from build123d import *

# Parameters (mm, degrees)
F0_W     = 48.26
F0_H     = 45.72
F0_R     = 1.397
F0_R_2   = 3.175
F1_DEPTH = 60.96
F2_DEPTH = 12.7
F3_DEPTH = 7.62


with BuildPart() as f1:
    # F0 (on Top) → F1 (new body)
    with BuildSketch(Plane.XY):
        Rectangle(F0_W, F0_H)
        with Locations((-17.145, -15.875)):
            Circle(F0_R, mode=Mode.SUBTRACT)
        with Locations((0, -15.875)):
            Circle(F0_R_2, mode=Mode.SUBTRACT)
        with Locations((17.145, -15.875)):
            Circle(F0_R, mode=Mode.SUBTRACT)
        with Locations((-17.145, 15.875)):
            Circle(F0_R, mode=Mode.SUBTRACT)
        with Locations((0, 15.875)):
            Circle(F0_R_2, mode=Mode.SUBTRACT)
        with Locations((17.145, 15.875)):
            Circle(F0_R, mode=Mode.SUBTRACT)
        with Locations((0, 15.875)):
            Circle(F0_R_2)
        with Locations((0, -15.875)):
            Circle(F0_R_2)
        with Locations((-17.145, 15.875)):
            Circle(F0_R)
        with Locations((-17.145, -15.875)):
            Circle(F0_R)
        with Locations((17.145, 15.875)):
            Circle(F0_R)
        with Locations((17.145, -15.875)):
            Circle(F0_R)
    extrude(amount=-F1_DEPTH)

    # F0 (on Top) → F2 (cut)
    with BuildSketch(Plane.XY):
        with Locations((-17.145, 15.875)):
            Circle(F0_R)
        with Locations((-17.145, -15.875)):
            Circle(F0_R)
        with Locations((17.145, 15.875)):
            Circle(F0_R)
        with Locations((17.145, -15.875)):
            Circle(F0_R)
    extrude(amount=-F2_DEPTH, mode=Mode.SUBTRACT)

    # F0 (on Top) → F3 (join)
    with BuildSketch(Plane.XY):
        with Locations((0, 15.875)):
            Circle(F0_R_2)
        with Locations((0, -15.875)):
            Circle(F0_R_2)
    extrude(amount=F3_DEPTH)


solid = f1.part
Read the model definition and answer for the solid it produces. Units are mm, in the model's axes. A direction names the side the tool comes from. Coordinates: 2 decimals unless noted, no trailing zeros. Loops run counter-clockwise (first coordinate to the right, second up) from the corner with the lowest first, then second, coordinate; pieces in that order, holes last.
Q1. The part is cut by section B-B on y = 6. Write down the section's boundary in (x, z).
Q2. The part is cut by section A-A on x = 0. Write down the section's boundary in (y, z).
Q3. The mould has two halves that part along X. Classify faces 1 (the face through (-24.13, 0, -30)), 2 (the face through (0, -16, 7.62)), 3 (the face through (17, -16, -12.7)): +X half, -X half, draft (parallel to the pull), parting line (faces both ways), or undercut.
Q4. Consider probe 1 along Z at (x, y) = (17, -14); probe 2 along X at (y, z) = (13, 1.5). Determine where each line is inside the solid, lowest interval first.
Q5. Each of these flat-tipped pins is pushed along its axis until it touches: pin 1 Ø6 at (x, y) = (-9.5, -5.5) entering from +Z; pin 2 Ø0.8 at (x, y) = (17, -15.5) entering from +Z. Where does it stop, or does it pass through?
Q6. Which of the six approach directions +Z, -Z, +X, -X, +Y, -Y give full straight-line access (tool end or side, diameter ignored) to faces 4 (the face through (0, 16, 7.62)), 5 (the face through (-0.413, 19.023, 3.757))?
Q7. The part is cut by section C-C on x = -10.5. Write down the section's boundary in (y, z).
Results below:
1. outline: (-24.13, -60.96) - (24.13, -60.96) - (24.13, 0) - (-24.13, 0) - close
2. outline: (-22.86, -60.96) - (22.86, -60.96) - (22.86, 0) - (19.05, 0) - (19.05, 7.62) - (12.7, 7.62) - (12.7, 0) - (-12.7, 0) - (-12.7, 7.62) - (-19.05, 7.62) - (-19.05, 0) - (-22.86, 0) - close
3. face 1: -X half
3. face 2: draft
3. face 3: undercut
4. probe 1: z = -60.96 to 0
4. probe 2: x = -1.35 to 1.35
5. pin 1: stops at z = 0
5. pin 2: stops at z = -12.7
6. face 4: +Z, +X, -X, +Y, -Y
6. face 5: +Z
7. outline: (-22.86, -60.96) - (22.86, -60.96) - (22.86, 0) - (-22.86, 0) - close
